Build history of the part. All positions in model axes, mm. Face numbers are marked on the shaded views. A direction names the side the tool comes from. Round coordinates to 2 decimals unless told otherwise and drop trailing zeros. Write each loop counter-clockwise with the first axis right and the second up, starting at its lowest first coordinate (ties: lowest second). Pieces come first, ordered by that corner, then holes.
1) Wall check: probe 1 along Y at (x, z) = (1.05, 0); probe 2 along Y at (x, z) = (0.45, 0); probe 3 along Z at (x, y) = (1.2, 3.5). Give the ranges that are in metal, low to high.
2) Which spindle directions (+Z, -Z, +X, -X, +Y, -Y) get a long thin tool onto all of the face, cutting with end or side? Do the marked faces 4 and 5. Say none if no direction does.
3) Saw through at A-A (y = 0). Write the cut outline in (x, z).
4) Saw through at C-C (x = 2.05). Write the cut outline in (y, z), plus the area to 3 significant figures.
5) Saw through at B-B (z = -3.5). Write the cut outline in (x, y), plus the area to 3 significant figures.
6) Pull direction Z, two halves, no side cores. Call the marked faces 1, 2 and 3: +Z half, -Z half, draft (parallel to the pull), parting line (faces both ways), or undercut.
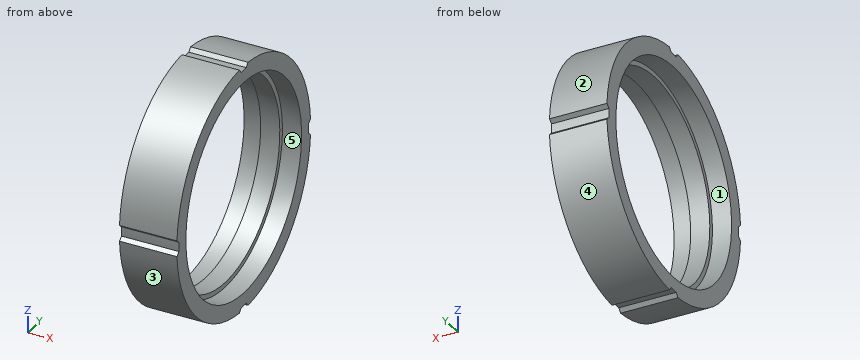
from build123d import *

# Parameters (mm, degrees)
EXTRUS_O4_DEPTH       = 8.668441823
PADR_OCIRCULAR2_COUNT = 4


with BuildPart() as part:
    # Esboço4 → Revolução1 (revolve)
    with BuildSketch(Plane.YX, mode=Mode.PRIVATE) as revolu_o1_sk:
        Polygon((-5.15, -0.116989073), (-5.15, 2.283010927), (-4.45, 2.283010927), (-4.45, 1.483010927), (-4.25, 1.483010927), (-4.25, 0.683010927), (-4.45, 0.683010927), (-4.45, -0.116989073), align=None)
    revolve(revolu_o1_sk.sketch.rotate(Axis((-0.622453524, 0, 0), (1, 0, 0)), 270), axis=Axis((-0.622453524, 0, 0), (1, 0, 0)))

    # Esboço5 → Extrusão4 (cut, through all)
    with BuildSketch(Plane(origin=(2.283010927, 0, 0), x_dir=(0, 0, 1), z_dir=(1, 0, 0))):
        with BuildLine():
            Line((-0.196837681, 4.979857893), (-0.332878645, 5.139230663))
            ThreePointArc((-0.332878645, 5.139230663), (0, 5.15), (0.332878645, 5.139230663))
            Line((0.332878645, 5.139230663), (0.196837681, 4.979857893))
            ThreePointArc((0.196837681, 4.979857893), (0, 4.983746554), (-0.196837681, 4.979857893))
        make_face()
    extrus_o4 = extrude(amount=-EXTRUS_O4_DEPTH, mode=Mode.SUBTRACT)

    # PadrãoCircular2: Extrusão4 ×4 about axis
    padr_ocircular2_axis = Axis((0, 0, 0), (1, 0, 0))
    for i in range(1, PADR_OCIRCULAR2_COUNT):
        add(extrus_o4.rotate(padr_ocircular2_axis, i * 360 / PADR_OCIRCULAR2_COUNT), mode=Mode.SUBTRACT)


solid = part.part
Evaluation:
1. probe 1: y = -4.98 to -4.25, 4.25 to 4.98
1. probe 2: y = -4.98 to -4.45, 4.45 to 4.98
1. probe 3: z = -3.78 to -2.41, 2.41 to 3.78
2. face 4: -Z, +X, -X, +Y
2. face 5: +X
3. outline: (-0.12, -4.98) - (2.28, -4.98) - (2.28, -4.45) - (1.48, -4.45) - (1.48, -4.25) - (0.68, -4.25) - (0.68, -4.45) - (-0.12, -4.45) - close; (-0.12, 4.45) - (0.68, 4.45) - (0.68, 4.25) - (1.48, 4.25) - (1.48, 4.45) - (2.28, 4.45) - (2.28, 4.98) - (-0.12, 4.98) - close
4. outline: (-5.14, -0.33) arc R5.15 ccw to (-0.33, -5.14) - (-0.2, -4.98) arc R4.98 ccw to (0.2, -4.98) - (0.33, -5.14) arc R5.15 ccw to (5.14, -0.33) - (4.98, -0.2) arc R4.98 ccw to (4.98, 0.2) - (5.14, 0.33) arc R5.15 ccw to (0.33, 5.14) - (0.2, 4.98) arc R4.98 ccw to (-0.2, 4.98) - (-0.33, 5.14) arc R5.15 ccw to (-5.14, 0.33) - (-4.98, 0.2) arc R4.98 ccw to (-4.98, -0.2) - close; hole circle Ø8.9 at (0, 0)
4. area: 20.8 mm2
5. outline: (-0.12, -3.78) - (2.28, -3.78) - (2.28, -2.75) - (1.48, -2.75) - (1.48, -2.41) - (0.68, -2.41) - (0.68, -2.75) - (-0.12, -2.75) - close; (-0.12, 2.75) - (0.68, 2.75) - (0.68, 2.41) - (1.48, 2.41) - (1.48, 2.75) - (2.28, 2.75) - (2.28, 3.78) - (-0.12, 3.78) - close
5. area: 5.48 mm2
6. face 1: undercut
6. face 2: +Z half
6. face 3: -Z half
